```python
from build123d import *

# Parameters (mm, degrees)
SKETCH_1_R               = 4.05
EXTRUDE_1_DEPTH          = 10
SKETCH_2_W               = 16
SKETCH_2_H               = 27.984210489
EXTRUDE_2_DEPTH          = 5
SKETCH_3_R               = 2.3
CUT_EXTRUDE_1_DEPTH      = 5
CHAMFER_2_SIZE           = 5
CHAMFER_3_SIZE           = 10
CHAMFER_3_SIZE2          = 5.773502692
EXTRUDE_3_DEPTH          = 3
CHAMFER_5_SIZE           = 5
CHAMFER_6_SIZE           = 5
FILLET_1_R               = 8
CUT_EXTRUDE_3_DEPTH      = 20
CUT_EXTRUDE_3_DEPTH_BACK = 4
SKETCH_7_W               = 3.5
SKETCH_7_H               = 100.709566722
EXTRUDE_4_DEPTH          = 2
EXTRUDE_4_DEPTH_BACK     = 2
SKETCH_8_R               = 4.05
SKETCH_8_R_2             = 3
FILLET_2_R               = 0.5


with BuildPart() as part:
    # 草图1 → 凸台-拉伸1 (new body)
    with BuildSketch(Plane.XY):
        Polygon((-8, -77.5), (8, -77.5), (8, -61.5), (0, -54.489879842), (0, 35.510120158), (8, 42.5), (8, 57.5), (-8, 57.5), (-8, 42.5), (-8, -61.5), align=None)
        with Locations((0, -67.5)):
            Circle(SKETCH_1_R, mode=Mode.SUBTRACT)
    extrude(amount=EXTRUDE_1_DEPTH)

    # 草图2 → 凸台-拉伸2 (add)
    with BuildSketch(Plane.XY.offset(10)):
        with Locations((0, 65.211792125)):
            Rectangle(SKETCH_2_W, SKETCH_2_H)
    extrude(amount=EXTRUDE_2_DEPTH)

    # 草图3 → 切除-拉伸1 (cut)
    with BuildSketch(Plane.XY.offset(15)):
        with Locations((0, 66.5)):
            Circle(SKETCH_3_R)
    extrude(amount=-CUT_EXTRUDE_1_DEPTH, mode=Mode.SUBTRACT)

    # 倒角2
    chamfer_2_edges = [part.edges().sort_by_distance(p)[0] for p in [
        (0, 51.21968688, 10),
    ]]
    chamfer(chamfer_2_edges, length=CHAMFER_2_SIZE - 0.0001)  # a hair under: the kernel refuses the full size

    # 倒角3
    chamfer_3_edges = [part.edges().sort_by_distance(p)[0] for p in [
        (0, 57.5, 0),
    ]]
    chamfer_3_side = [part.faces().sort_by_distance(p)[0] for p in [
        (-2.385544593, -8.070394636, 0),
    ]]
    chamfer(chamfer_3_edges, length=CHAMFER_3_SIZE, length2=CHAMFER_3_SIZE2, reference=chamfer_3_side[0])

    # 草图5 → 凸台-拉伸3 (add)
    with BuildSketch(Plane(origin=(8, 0, 0), x_dir=(0, 0, -1), z_dir=(1, 0, 0))):
        Polygon((-10, 61.5), (-5.773502692, 57.5), (-10, 57.5), align=None)
    extrude_3 = extrude(amount=-EXTRUDE_3_DEPTH)

    # 镜向1: 凸台-拉伸3 across plane
    add(extrude_3.mirror(Plane(origin=(0, 0, 0), x_dir=(0, 0, 1), z_dir=(1, 0, 0))))

    # 倒角5
    chamfer_5_edges = [part.edges().sort_by_distance(p)[0] for p in [
        (-8, 79.203897369, 12.5),
        (8, 79.203897369, 12.5),
    ]]
    chamfer(chamfer_5_edges, length=CHAMFER_5_SIZE)

    # 倒角6
    chamfer_6_edges = [part.edges().sort_by_distance(p)[0] for p in [
        (-8, -77.5, 5),
    ]]
    chamfer(chamfer_6_edges, length=CHAMFER_6_SIZE)

    # 圆角1
    fillet_1_edges = [part.edges().sort_by_distance(p)[0] for p in [
        (8, -77.5, 5),
    ]]
    fillet(fillet_1_edges, radius=FILLET_1_R)

    # 草图7 → 切除-拉伸3 (cut, two sides: drawn at the far end of the back side and taken through both)
    with BuildSketch(Plane(origin=(0, 0, 0), x_dir=(0, 0, -1), z_dir=(1, 0, 0)).offset(-CUT_EXTRUDE_3_DEPTH_BACK)):
        with Locations((-1.75, -4.135096481)):
            Rectangle(SKETCH_7_W, SKETCH_7_H)
        with Locations((-8.25, -4.135096481)):
            Rectangle(SKETCH_7_W, SKETCH_7_H)
    extrude(amount=CUT_EXTRUDE_3_DEPTH + CUT_EXTRUDE_3_DEPTH_BACK, mode=Mode.SUBTRACT)

    # 草图8 → 凸台-拉伸4 (add, two sides: drawn at the far end of the back side and taken through both)
    with BuildSketch(Plane.XY.offset(5).offset(-EXTRUDE_4_DEPTH_BACK)):
        with Locations((0, -67.5)):
            Circle(SKETCH_8_R)
        with Locations((0, -67.5)):
            Circle(SKETCH_8_R_2, mode=Mode.SUBTRACT)
    extrude(amount=EXTRUDE_4_DEPTH + EXTRUDE_4_DEPTH_BACK)

    # 圆角2
    fillet_2_edges = [part.edges().sort_by_distance(p)[0] for p in [
        (-4.05, -67.5, 0),
        (-4.05, -67.5, 10),
    ]]
    fillet(fillet_2_edges, radius=FILLET_2_R)


solid = part.part
```
Can you work these out from the model? Positions are in its coordinate system, mm. A direction names the side the tool comes from. Coordinates: 2 decimals unless noted, no trailing zeros. Loops run counter-clockwise (first coordinate to the right, second up) from the corner with the lowest first, then second, coordinate; pieces in that order, holes last. Notation, with made-up numbers: (53, 75) -> (99, 75) arc R26 cw to (99, 110) -> close; hole circle Ø4 at (24, -24.5). An arc over 180 degrees is marked (long way). Answer as a JSON object with one key per item and string values.
1) Thinking about a two-plate mould opening in X: for faces 5 (the face through (-5, 59, 9)), 6 (the face through (8, -66, 5)), 7 (the face through (-2, 6, 3.5)), which applies, pulls with the +X half, pulls with the -X half, needs draft (parallel to the pull), parting line crosses it, or undercut?
Results:
{"face 5": "undercut", "face 6": "pulls with the +X half", "face 7": "needs draft"}
2) Imagine slicing it at D-D (y = 66.5). Please give me the cut outline in (x, z).
Results:
{"outline": "(-8, 10) -> (-2.3, 10) -> (-2.3, 15) -> (-8, 15) -> close; (2.3, 10) -> (8, 10) -> (8, 15) -> (2.3, 15) -> close"}
3) For faces 1 (the face through (0, -64, 3)), 2 (the face through (-2, -54.49, 8)), 3 (the face through (0, 57.5, 8)), 4 (the face through (-0.527, -63.484, 8.232)), which set-ups out of +Z, -Z, +X, -X, +Y, -Y let a thin tool reach every point of the face, with its end or its side?
Results:
{"face 1": "-Z", "face 2": "+Z, +X", "face 3": "-Z, +Y", "face 4": "+Z"}
4) If I drill on line 1 (Z direction, x = -7, y = 62.5); line 2 (Y direction, x = 2.5, z = 6.75); line 3 (Z direction, x = -6.75, y = 3.5), over which ranges is the centre line in solid material (lowest first)?
Results:
{"line 1": "z = 10 to 15", "line 2": "y = -77.1 to -69.16, -65.84 to -56.68, 46.22 to 57.5", "line 3": "z = 0 to 10"}
5) Imagine slicing it at A-A (y = -67.5). Please give me the cut outline in (x, z), then the cut area to 3 significant figures.
Results:
{"outline": "(-8, 0) -> (-4.55, 0) arc R0.5 ccw to (-4.05, 0.5) -> (-4.05, 3) -> (-3, 3) -> (-3, 7) -> (-4.05, 7) -> (-4.05, 9.5) arc R0.5 ccw to (-4.55, 10) -> (-8, 10) -> close; (3, 3) -> (4.05, 3) -> (4.05, 0.5) arc R0.5 ccw to (4.55, 0) -> (8, 0) -> (8, 10) -> (4.55, 10) arc R0.5 ccw to (4.05, 9.5) -> (4.05, 7) -> (3, 7) -> close", "area": "87.2 mm^2"}
6) For P1, Ø7.5, axis at x = 0, y = -67.5, coming from the -Z side; P2, Ø3, axis at x = -1.5, y = -14, coming from the +Z side; P3, Ø5, axis at x = 3, y = 68.5, coming from the -Z side, each with a flat end and sliding along its axis, tell me the tip position at first contact or that it passes through.
Results:
{"P1": "stops at z = 3", "P2": "stops at z = 6.5", "P3": "stops at z = 10"}
7) Imagine slicing it at B-B (z = 13.5). Please give me the cut outline in (x, y).
Results:
{"outline": "(-8, 49.72) -> (8, 49.72) -> (8, 74.2) -> (3, 79.2) -> (-3, 79.2) -> (-8, 74.2) -> close; hole circle Ø4.6 at (0, 66.5)"}
8) Imagine slicing it at C-C (y = 18). Please give me the cut outline in (x, z).
Results:
{"outline": "(-8, 0) -> (-4, 0) -> (-4, 3.5) -> (0, 3.5) -> (0, 6.5) -> (-4, 6.5) -> (-4, 10) -> (-8, 10) -> close"}
